Verification items for the finished model (mm, model axes). Face numbers are marked on the shaded views. Round coordinates to 2 decimals unless told otherwise and drop trailing zeros. Order: outer loops, then holes, each group sorted by start corner. A loop starts at its lowest first (then second) coordinate and runs counter-clockwise, first axis right, second up. Notation, with made-up numbers: M -17.75,34 L 32.25,34 A23 cw 32.25,53 Z; hole C 47.25,87 d9. An arc over 180 degrees is marked long. Answer as a JSON object with one key per item and string values. Group by question number.
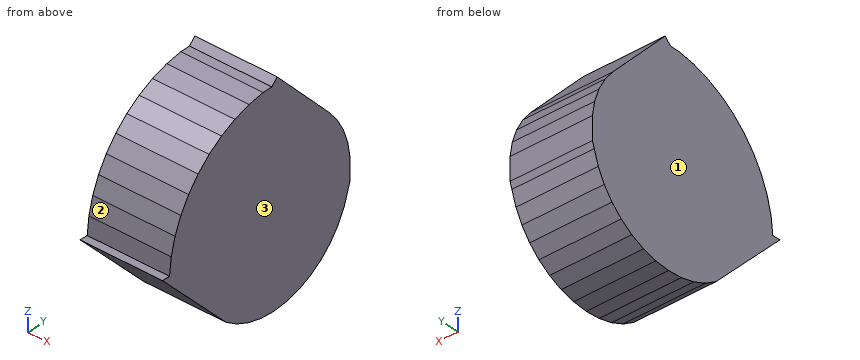
```python
from build123d import *

# Parameters (mm, degrees)
F1_DEPTH = 7


with BuildPart() as f1:
    # F0 (on Right) → F1 (new body)
    with BuildSketch(Plane.YZ):
        Polygon((-10.270449, -0.400699), (-4.092179, -6.819432), (-3.047954, -7.485725), (-1.908302, -7.971057), (-0.704311, -8.262191), (0.531178, -8.351182), (1.764465, -8.235605), (2.961906, -7.918611), (4.090843, -7.408849), (5.120478, -6.720222), (6.022723, -5.871515), (6.772974, -4.88588), (7.350761, -3.790199), (7.740323, -2.614362), (7.917699, -2.078977), (7.917699, -0.151823), (7.700671, 1.067708), (7.285879, 2.234883), (6.684631, 3.317867), (5.913329, 4.287119), (0.855827, 9.663673), (0.340538, 9.148384), (-0.500703, 9.148384), (-1.864732, 8.917333), (-3.241889, 8.484291), (-4.542701, 7.858209), (-5.74027, 7.052034), (-6.809833, 6.082434), (-7.729276, 4.969459), (-8.479586, 3.736121), (-9.045251, 2.407921), (-9.414573, 1.012325), (-9.579916, -0.421813), align=None)
    extrude(amount=F1_DEPTH)


solid = f1.part
```
Q1. Cross-section at C-C, the plane z = 6.5. Record the cut outline in (x, y).
Q2. Thickness scan on line 1 (Y direction, x = 1.75, z = -4.25); line 2 (Z direction, x = 4.5, y = -2); line 3 (Y direction, x = 0.75, z = -1). Record the ranges inside material, lowest first. Write a range as from..to.
Q3. Cross-section at B-B, the plane y = -6. Record the cut outline in (x, z), then the cut area to 3 significant figures.
Q4. Gauge pin test, flat ends, axial feed: pin 1 Ø4 at (x, z) = (6, 6) entering from -Y; pin 2 Ø2 at (x, y) = (4.5, 2.5) entering from -Z; pin 3 Ø1.5 at (x, z) = (1.5, 2) entering from +Y. Record the tip position at first contact, or that the pin passes through.
Q5. Release check for a two-part mould opening along X. For the marked faces 1, 2 and 3 record: released by +X, released by -X, zero draft, split by the parting line, or undercut.
Conclusion:
{
 "1": {"outline": "M 0,-6.35 L 7,-6.35 L 7,3.83 L 0,3.83 Z"},
 "2": {"line 1": "-6.57..7.11", "line 2": "-7.93..8.87", "line 3": "-9.69..7.92"},
 "3": {"outline": "M 0,-4.84 L 7,-4.84 L 7,6.82 L 0,6.82 Z", "area": "81.6 mm2"},
 "4": {"pin 1": "y = -8.32", "pin 2": "z = -8.26", "pin 3": "y = 7.64"},
 "5": {"face 1": "released by -X", "face 2": "zero draft", "face 3": "released by +X"}
}
